Here's how the part is built. I have some questions about the finished solid (model axes, mm). A direction names the side the tool comes from. Coordinates: 2 decimals unless noted, no trailing zeros. Write each loop counter-clockwise with the first axis right and the second up, starting at its lowest first coordinate (ties: lowest second). Pieces come first, ordered by that corner, then holes. Notation, with made-up numbers: (36, -36.75) -> (57, -36.75) arc R17 cw to (57, -31.75) -> close; hole circle Ø4 at (-4.5, -13.75). An arc over 180 degrees is marked (long way). Put each result on its own line as item: value.
```python
from build123d import *

# Parameters (mm, degrees)
F1_DEPTH = 5.5
F2_DEPTH = 15.5
F3_R     = 1.7


with BuildPart() as f1:
    # F0 (on Top) → F1 (new body)
    with BuildSketch(Plane.XY):
        with BuildLine():
            add(Edge.make_bspline(
                [(-29.498119845, 0), (-29.6541738862, 14.1305088281), (-27.4827572547, 20.9253169468), (-19.6571877436, 24.5), (-16.598119845, 24.5)],
                knots=[0, 0, 0, 0, 0.3045466279, 0.5, 0.5, 0.5, 0.5], degree=3))
            Line((-29.498119845, 0), (-26.7035992752, 2.7945205698))
            ThreePointArc((-26.7035992752, 2.7945205698), (-26.6666227292, 5.4435028843), (-24.0176404147, 5.4804794302))
            Line((-24.0176404147, 5.4804794302), (-16.598119845, 12.9))
            Line((-16.598119845, 12.9), (-16.598119845, 18.6))
            ThreePointArc((-16.598119845, 18.6), (-18.498119845, 20.5), (-16.598119845, 22.4))
            Line((-16.598119845, 22.4), (-16.598119845, 24.5))
        make_face()
        with BuildLine():
            add(Edge.make_bspline(
                [(-16.598119845, 24.5), (-13.5390519463, 24.5), (-10.4799840477, 23.1026322863), (-8.2849164094, 21.2132034356)],
                knots=[0.5, 0.5, 0.5, 0.5, 0.6954533721, 0.6954533721, 0.6954533721, 0.6954533721], degree=3))
            Line((-16.598119845, 24.5), (-16.598119845, 22.4))
            ThreePointArc((-16.598119845, 22.4), (-15.2546169607, 21.8435028843), (-14.698119845, 20.5))
            ThreePointArc((-14.698119845, 20.5), (-15.2546169607, 19.1564971157), (-16.598119845, 18.6))
            Line((-16.598119845, 18.6), (-16.598119845, 12.9))
            Line((-16.598119845, 12.9), (-8.2849164094, 21.2132034356))
        make_face()
        with BuildLine():
            ThreePointArc((-14.698119845, 20.5), (-15.2546169607, 21.8435028843), (-16.598119845, 22.4))
            Line((-16.598119845, 22.4), (-16.598119845, 20.5))
            Line((-16.598119845, 20.5), (-16.598119845, 18.6))
            ThreePointArc((-16.598119845, 18.6), (-15.2546169607, 19.1564971157), (-14.698119845, 20.5))
        make_face()
        with BuildLine():
            Line((-16.598119845, 20.5), (-16.598119845, 22.4))
            ThreePointArc((-16.598119845, 22.4), (-18.498119845, 20.5), (-16.598119845, 18.6))
            Line((-16.598119845, 18.6), (-16.598119845, 20.5))
        make_face()
        with BuildLine():
            Line((-16.598119845, 4.1), (-16.598119845, 0))
            Line((-16.598119845, 0), (-3.698119845, 0))
            add(Edge.make_bspline(
                [(-8.2849164094, 21.2132034356), (-4.8646610296, 18.269180628), (-3.5420658037, 14.1305088281), (-3.698119845, 0)],
                knots=[0.6954533721, 0.6954533721, 0.6954533721, 0.6954533721, 1, 1, 1, 1], degree=3))
            Line((-8.2849164094, 21.2132034356), (-16.598119845, 12.9))
            Line((-16.598119845, 12.9), (-16.598119845, 4.1))
        make_face()
        with BuildLine():
            ThreePointArc((-5.973119845, 4.1), (-7.873119845, 2.2), (-9.773119845, 4.1))
            ThreePointArc((-9.773119845, 4.1), (-7.873119845, 6), (-5.973119845, 4.1))
        make_face(mode=Mode.SUBTRACT)
        with BuildLine():
            ThreePointArc((-5.973119845, 4.1), (-7.873119845, 6), (-9.773119845, 4.1))
            ThreePointArc((-9.773119845, 4.1), (-7.873119845, 2.2), (-5.973119845, 4.1))
        make_face()
        with BuildLine():
            Line((-23.423119845, 4.1), (-16.598119845, 4.1))
            Line((-16.598119845, 4.1), (-16.598119845, 12.9))
            Line((-16.598119845, 12.9), (-24.0176404147, 5.4804794302))
            ThreePointArc((-24.0176404147, 5.4804794302), (-23.5780681384, 4.8515281374), (-23.423119845, 4.1))
        make_face()
        with BuildLine():
            Line((-26.7035992752, 2.7945205698), (-29.498119845, 0))
            Line((-29.498119845, 0), (-16.598119845, 0))
            Line((-16.598119845, 0), (-16.598119845, 4.1))
            Line((-16.598119845, 4.1), (-23.423119845, 4.1))
            ThreePointArc((-23.423119845, 4.1), (-24.6205925919, 2.3346514625), (-26.7035992752, 2.7945205698))
        make_face()
        with BuildLine():
            Line((-24.0176404147, 5.4804794302), (-26.7035992752, 2.7945205698))
            ThreePointArc((-26.7035992752, 2.7945205698), (-24.6205925919, 2.3346514625), (-23.423119845, 4.1))
            ThreePointArc((-23.423119845, 4.1), (-23.5780681384, 4.8515281374), (-24.0176404147, 5.4804794302))
        make_face()
        with BuildLine():
            ThreePointArc((-24.0176404147, 5.4804794302), (-26.6666227292, 5.4435028843), (-26.7035992752, 2.7945205698))
            Line((-26.7035992752, 2.7945205698), (-24.0176404147, 5.4804794302))
        make_face()
    extrude(amount=F1_DEPTH)

    # F0 (on Top) → F2 (join)
    with BuildSketch(Plane.XY):
        with BuildLine():
            ThreePointArc((-24.0176404147, 5.4804794302), (-26.6666227292, 5.4435028843), (-26.7035992752, 2.7945205698))
            Line((-26.7035992752, 2.7945205698), (-24.0176404147, 5.4804794302))
        make_face()
        with BuildLine():
            Line((-24.0176404147, 5.4804794302), (-26.7035992752, 2.7945205698))
            ThreePointArc((-26.7035992752, 2.7945205698), (-24.6205925919, 2.3346514625), (-23.423119845, 4.1))
            ThreePointArc((-23.423119845, 4.1), (-23.5780681384, 4.8515281374), (-24.0176404147, 5.4804794302))
        make_face()
        with BuildLine():
            ThreePointArc((-14.698119845, 20.5), (-15.2546169607, 21.8435028843), (-16.598119845, 22.4))
            Line((-16.598119845, 22.4), (-16.598119845, 20.5))
            Line((-16.598119845, 20.5), (-16.598119845, 18.6))
            ThreePointArc((-16.598119845, 18.6), (-15.2546169607, 19.1564971157), (-14.698119845, 20.5))
        make_face()
        with BuildLine():
            Line((-16.598119845, 20.5), (-16.598119845, 22.4))
            ThreePointArc((-16.598119845, 22.4), (-18.498119845, 20.5), (-16.598119845, 18.6))
            Line((-16.598119845, 18.6), (-16.598119845, 20.5))
        make_face()
        with BuildLine():
            ThreePointArc((-5.973119845, 4.1), (-7.873119845, 6), (-9.773119845, 4.1))
            ThreePointArc((-9.773119845, 4.1), (-7.873119845, 2.2), (-5.973119845, 4.1))
        make_face()
    extrude(amount=F2_DEPTH)

    # F3
    f3_edges = [f1.edges().sort_by_distance(p)[0] for p in [
        (-16.59812, 18.6, 15.5),
        (-23.94264, 5.405479, 15.5),
        (-5.97312, 4.1, 15.5),
    ]]
    fillet(f3_edges, radius=F3_R)


solid = f1.part
```
Item 1: For P1, Ø1.5, axis at x = -7.5, y = 15, coming from the +Z side; P2, Ø3, axis at x = -24.5, z = 9, coming from the -Y side; P3, Ø1, axis at y = 11, z = 5.5, coming from the +X side, each with a flat end and sliding along its axis, tell me the tip position at first contact or that it passes through.
Output:
P1: stops at z = 5.5
P2: stops at y = 2.2
P3: stops at x = -4
Item 2: If we mould it in two halves opening along X, with no side actions, what happens to faces 3 (the flat face through (-17, 10, 0)), 4 (the cylindrical face through (-8.75, 5.786, 9.592))? For each: released by +X, released by -X, zero draft, split by the parting line, or undercut.
Output:
face 3: zero draft
face 4: undercut
Item 3: Imagine slicing it at A-A on z = 9.5. Write out the boundary of the cut face in (x, y), then the cut area to 3 significant figures.
Output:
outline: circle Ø3.8 at (-25.32, 4.1); circle Ø3.8 at (-16.6, 20.5); circle Ø3.8 at (-7.87, 4.1)
area: 34.0 mm²
Item 4: Which directions (+Z, -Z, +X, -X, +Y, -Y) give clear straight access to the entire face, cutting with the end or side of a thin tool? Please do faces 1 (the flat face through (-16, 10, 5.5)), 2 (the flat face through (-17, 0, 3)).
Output:
face 1: +Z
face 2: +Z, -Z, +X, -X, -Y
Item 5: Please list where these lines run through material, in increasing order: line 1 along Z through (x, y) = (-19.5, 1.5); line 2 along Y through (x, z) = (-16.5, 5); line 3 along X through (y, z) = (5, 13.5). Write a range as from..to.
Output:
line 1: z = 0..5.5
line 2: y = 0..24.5
line 3: x = -27..-23.65, -9.55..-6.2
